Check sheet for the drawn part. Datum: minimum x, y, z corner. Units: mm. A direction names the side the tool comes from. Round coordinates to 2 decimals unless told otherwise and drop trailing zeros. Loops run counter-clockwise (first coordinate to the right, second up) from the corner with the lowest first, then second, coordinate; pieces in that order, holes last.
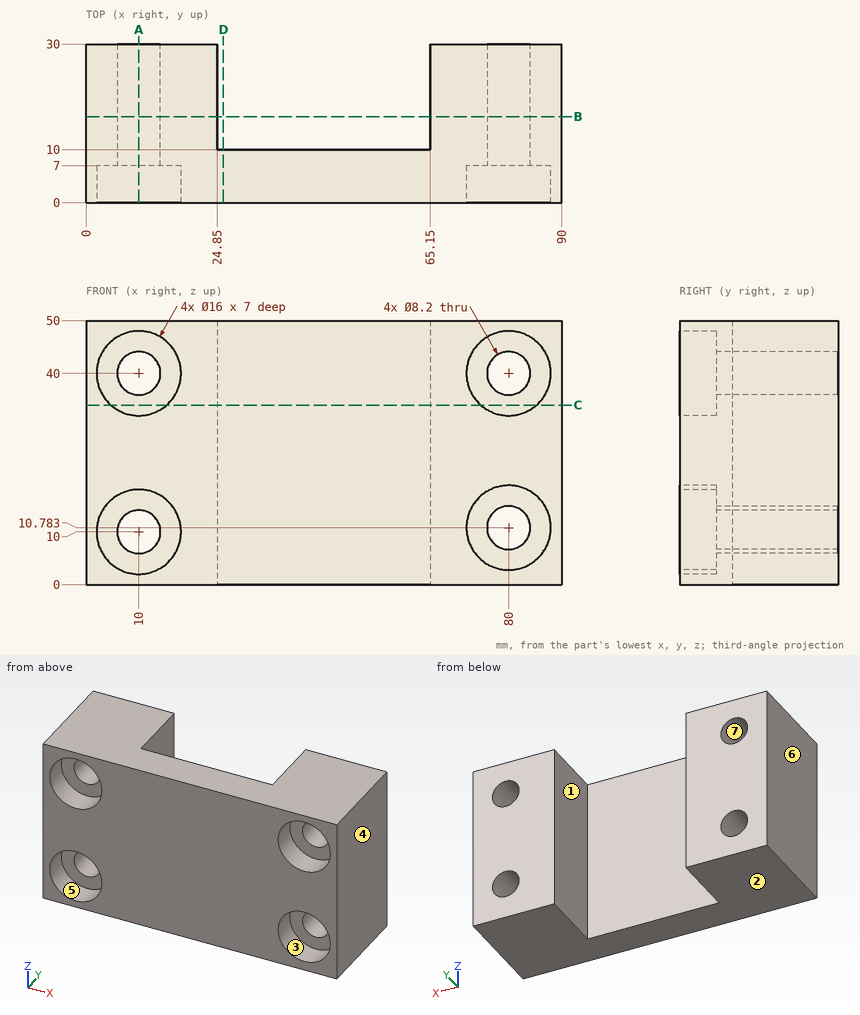
1) Sectioned sample at C-C, the plane z = 34. Record the cut outline in (x, y).
Report:
outline: (0, 0) - (4.71, 0) - (4.71, 7) - (15.29, 7) - (15.29, 0) - (74.71, 0) - (74.71, 7) - (85.29, 7) - (85.29, 0) - (90, 0) - (90, 30) - (65.15, 30) - (65.15, 10) - (24.85, 10) - (24.85, 30) - (0, 30) - close
2) Sectioned sample at B-B, the plane y = 16.25. Record the cut outline in (x, z), then the cut area to 3 significant figures.
Report:
outline: (0, 0) - (24.85, 0) - (24.85, 50) - (0, 50) - close; (65.15, 0) - (90, 0) - (90, 50) - (65.15, 50) - close; hole circle Ø8.2 at (10, 10); hole circle Ø8.2 at (10, 40); hole circle Ø8.2 at (80, 10.78); hole circle Ø8.2 at (80, 40)
area: 2,270 mm2
3) Gauge pin test, flat ends, axial feed: pin 1 (21 mm diameter, centred on x = 80, z = 40, fed in from +Y); pin 2 (8 mm diameter, centred on x = 78, z = 8.5, fed in from -Y); pin 3 (5 mm diameter, centred on x = 80, z = 10.78, fed in from -Y); pin 4 (10 mm diameter, centred on x = 33.5, z = 15, fed in from +Y). Record the tip position at first contact, or that the pin passes through.
Report:
pin 1: stops at y = 30
pin 2: stops at y = 7
pin 3: passes through
pin 4: stops at y = 10
4) Sectioned sample at D-D, the plane x = 26. Record the cut outline in (y, z), then the cut area to 3 significant figures.
Report:
outline: (0, 0) - (10, 0) - (10, 50) - (0, 50) - close
area: 500 mm2
5) Scan lines: line 1 along Z through (x, y) = (80, 2.75); line 2 along Z through (x, y) = (10, 4.5); line 3 along X through (y, z) = (24, 38). Record each from-to range of solid material in increasing order.
Report:
line 1: z = 0 to 2.78, 18.78 to 32, 48 to 50
line 2: z = 0 to 2, 18 to 32, 48 to 50
line 3: x = 0 to 6.42, 13.58 to 24.85, 65.15 to 76.42, 83.58 to 90
6) Mould release check, pull along X, two halves, no side actions. Record for the marked faces 4, 5, 6 and 7: +X half, -X half, draft (parallel to the pull), parting line (faces both ways), or undercut.
Report:
face 4: +X half
face 5: undercut
face 6: -X half
face 7: undercut
7) Sectioned sample at A-A, the plane x = 10. Record the cut outline in (y, z), then the cut area to 3 significant figures.
Report:
outline: (0, 0) - (30, 0) - (30, 5.9) - (7, 5.9) - (7, 2) - (0, 2) - close; (0, 18) - (7, 18) - (7, 14.1) - (30, 14.1) - (30, 35.9) - (7, 35.9) - (7, 32) - (0, 32) - close; (0, 48) - (7, 48) - (7, 44.1) - (30, 44.1) - (30, 50) - (0, 50) - close
area: 899 mm2
8) Access from +Z, -Z, +X, -X, +Y, -Y to the whole of each face (thin tool, end or side, straight path). Record for the marked faces 1, 2 and 3.
Report:
face 1: +Z, -Z, +Y
face 2: -Z, +X, -X, +Y, -Y
face 3: -Y
